Verification items for the finished model (mm, model axes). A direction names the side the tool comes from. Coordinates: 2 decimals unless noted, no trailing zeros. Order: outer loops, then holes, each group sorted by start corner. A loop starts at its lowest first (then second) coordinate and runs counter-clockwise, first axis right, second up. Notation, with made-up numbers: M 83,-19 L 121,-19 A21 cw 121,-7 Z; hole C -15,4.25 d8. An arc over 180 degrees is marked long. Return JSON: item names as keys, results as strings.
```python
from build123d import *

# Parameters (mm, degrees)
BOSS_EXTRUDE1_DEPTH = 5
FILLET1_R           = 10
BOSS_EXTRUDE2_DEPTH = 9.2
CUT_EXTRUDE1_DEPTH  = 3.2
SKETCH2_R           = 2.4999999999999996
SKETCH2_R_2         = 2.500000000000053
SKETCH2_R_3         = 2.5000000000000964
SKETCH2_R_4         = 2.5000000000000018
SKETCH2_R_5         = 2.4999999999999947
SKETCH2_R_6         = 14.287500000000001
CUT_EXTRUDE2_DEPTH  = 50.49730061393943
FILLET2_R           = 10


with BuildPart() as part:
    # Sketch1 → Boss-Extrude1 (new body)
    with BuildSketch(Plane(origin=(0, 0, 0), x_dir=(1, 0, 0), z_dir=(0, 1, 0))):
        Polygon((31.8, 18.359738560230117), (-9.39e-15, 36.719477120460205), (-31.799999999999994, 18.359738560230117), (-31.799999999999986, -18.359738560230095), (2.025e-14, -36.719477120460205), (31.800000000000008, -18.35973856023011), align=None)
    extrude(amount=BOSS_EXTRUDE1_DEPTH)

    # Fillet1
    fillet1_edges = [part.edges().sort_by_distance(p)[0] for p in [
        (31.800000000000008, 2.5, 18.35973856023011),
        (2.025e-14, 2.5, 36.719477120460205),
        (-31.799999999999986, 2.5, 18.359738560230095),
        (-31.799999999999994, 2.5, -18.359738560230117),
        (-9.39e-15, 2.5, -36.719477120460205),
        (31.8, 2.5, -18.359738560230117),
    ]]
    fillet(fillet1_edges, radius=FILLET1_R)

    # Sketch3 → Boss-Extrude2 (add)
    with BuildSketch(Plane.XZ):
        Polygon((27.499999999999996, 15.877132402714718), (9.57e-15, 31.754264805429415), (-27.500000000000004, 15.877132402714711), (-27.499999999999996, -15.877132402714711), (1.826e-14, -31.754264805429422), (27.50000000000001, -15.877132402714718), align=None)
    extrude(amount=BOSS_EXTRUDE2_DEPTH)

    # Sketch4 → Cut-Extrude1 (cut)
    with BuildSketch(Plane.XZ):
        Polygon((2.8499999999999854, -30.108816538239008), (4.199999999999984, -32.44708512845699), (26.000000000000007, -19.86084926012314), (24.650000000000006, -17.522580669905157), align=None)
        Polygon((-25.999999999999996, -19.860849260123146), (-4.200000000000003, -32.447085128456976), (-2.8499999999999983, -30.108816538238976), (-24.649999999999988, -17.52258066990515), align=None)
        Polygon((27.499999999999996, -12.586235868333851), (30.200000000000003, -12.586235868333851), (30.200000000000006, 12.586235868333848), (27.499999999999996, 12.586235868333848), align=None)
        Polygon((24.650000000000006, 17.522580669905146), (26.00000000000001, 19.860849260123135), (4.200000000000031, 32.44708512845697), (2.8500000000000263, 30.108816538238973), align=None)
        Polygon((-30.19999999999999, 12.58623586833384), (-30.199999999999996, -12.586235868333855), (-27.5, -12.58623586833386), (-27.500000000000004, 12.58623586833384), align=None)
        Polygon((-4.199999999999982, 32.44708512845697), (-25.99999999999999, 19.860849260123125), (-24.64999999999999, 17.52258066990515), (-2.849999999999986, 30.108816538238987), align=None)
    extrude(amount=-CUT_EXTRUDE1_DEPTH, mode=Mode.SUBTRACT)

    # Sketch2 → Cut-Extrude2 (cut, through all)
    with BuildSketch(Plane(origin=(0, 5, 0), x_dir=(1, 0, 0), z_dir=(0, 1, 0))):
        with Locations(Location((1.561e-14, 23.799999999999994, 0), (0, 0, 270))):
            Circle(SKETCH2_R)
        with Locations(Location((20.61140461006965, 11.899999999999997, 0), (0, 0, 270))):
            Circle(SKETCH2_R_2)
        with Locations(Location((20.61140461006965, -11.899999999999993, 0), (0, 0, 270))):
            Circle(SKETCH2_R_3)
        with Locations(Location((-1.561e-14, -23.800000000000015, 0), (0, 0, 270))):
            Circle(SKETCH2_R_4)
        with Locations(Location((-20.61140461006965, -11.899999999999993, 0), (0, 0, 270))):
            Circle(SKETCH2_R_5)
        with Locations(Location((-20.611404610069634, 11.899999999999999, 0), (0, 0, 270))):
            Circle(SKETCH2_R_5)
        with Locations(Location((0, 0, 0), (0, 0, 270))):
            Circle(SKETCH2_R_6)
    extrude(amount=-CUT_EXTRUDE2_DEPTH, mode=Mode.SUBTRACT)

    # Fillet2
    fillet2_edges = [part.edges().sort_by_distance(p)[0] for p in [
        (27.499999999999996, -4.6, 15.877132402714718),
        (9.57e-15, -4.6, 31.754264805429415),
        (-27.500000000000004, -4.6, 15.877132402714711),
        (-27.499999999999996, -4.6, -15.877132402714711),
        (27.50000000000001, -4.6, -15.877132402714718),
        (1.826e-14, -4.6, -31.754264805429422),
    ]]
    fillet(fillet2_edges, radius=FILLET2_R)


solid = part.part
```
Q1. Cross-section at D-D, the plane y = -3.5. Record the boundary of the cut face in (x, z) (1 decimal), and give its area (3 significant figures).
Values:
{"outline": "M -27.5,-10.1 A10 ccw -22.5,-18.8 L -5,-28.9 A10 ccw 5,-28.9 L 22.5,-18.8 A10 ccw 27.5,-10.1 L 27.5,10.1 A10 ccw 22.5,18.8 L 5,28.9 A10 ccw -5,28.9 L -22.5,18.8 A10 ccw -27.5,10.1 Z; hole C -20.6,-11.9 d5; hole C -20.6,11.9 d5; hole C 0,0 d28.6; hole C 0,-23.8 d5; hole C 0,23.8 d5; hole C 20.6,-11.9 d5; hole C 20.6,11.9 d5", "area": "1,830 mm^2"}
Q2. Cross-section at A-A, the plane x = 0. Record the boundary of the cut face in (y, z).
Values:
{"outline": "M -9.2,-30.21 L 0,-30.21 L 0,-35.17 L 5,-35.17 L 5,-26.3 L -9.2,-26.3 Z; M -9.2,-21.3 L 5,-21.3 L 5,-14.29 L -9.2,-14.29 Z; M -9.2,14.29 L 5,14.29 L 5,21.3 L -9.2,21.3 Z; M -9.2,26.3 L 5,26.3 L 5,35.17 L 0,35.17 L 0,30.21 L -9.2,30.21 Z"}
Q3. Material ranges on line 1 along X through (y, z) = (-4.25, -11.9); line 2 along Z through (x, y) = (-1, 2.5); line 3 along X through (y, z) = (-6.5, 0), recorded low to high.
Values:
{"line 1": "-27.34 to -23.11, -18.11 to -7.91, 7.91 to 18.11, 23.11 to 27.34", "line 2": "-35.12 to -26.09, -21.51 to -14.25, 14.25 to 21.51, 26.09 to 35.12", "line 3": "-27.5 to -14.29, 14.29 to 27.5"}
Q4. Go/stop test with flat-tipped pins: pin 1 (8 mm diameter, centred on y = 1.5, z = -27.5, fed in from +X); pin 2 (6 mm diameter, centred on x = -16, z = -27, fed in from -Y); pin 3 (4 mm diameter, centred on x = 25.5, y = 2, fed in from +Z). Record where each tip stops, or that it passes through.
Values:
{"pin 1": "x = 22.9", "pin 2": "y = 0", "pin 3": "z = 23.15"}
Q5. Cross-section at C-C, the plane x = -13. Record the boundary of the cut face in (y, z).
Values:
{"outline": "M -9.2,-24.25 L 3.2,-24.25 L 3.2,-27.37 L 0,-27.37 L 0,-29.21 L 5,-29.21 L 5,-5.93 L -9.2,-5.93 Z; M -9.2,5.93 L 5,5.93 L 5,29.21 L 0,29.21 L 0,27.37 L 3.2,27.37 L 3.2,24.25 L -9.2,24.25 Z"}
Q6. Draft check along Z on faces 3 (the face through (-14, 3.2, 25)), 4 (the face through (16.053, 2.465, -27.452)), 5 (the face through (15.747, 2.465, 27.628)). Enter one of: pulls with the +Z half, pulls with the -Z half, needs draft (parallel to the pull), parting line crosses it, or undercut.
Values:
{"face 3": "undercut", "face 4": "pulls with the -Z half", "face 5": "pulls with the +Z half"}
Q7. Cross-section at B-B, the plane z = 0. Record the boundary of the cut face in (x, y), and give its area (3 significant figures).
Values:
{"outline": "M -31.8,0 L -30.2,0 L -30.2,3.2 L -27.5,3.2 L -27.5,-9.2 L -14.29,-9.2 L -14.29,5 L -31.8,5 Z; M 14.29,-9.2 L 27.5,-9.2 L 27.5,3.2 L 30.2,3.2 L 30.2,0 L 31.8,0 L 31.8,5 L 14.29,5 Z", "area": "401 mm^2"}
Q8. Tool access check on faces 1 (the face through (-15.253, 1.578, -26.066)), 2 (the face through (-18.133, -2.001, 11.575)). Record the directions out of +Z, -Z, +X, -X, +Y, -Y that give a thin tool (end or side, any length) a straight path to the whole face; none if there is none.
Values:
{"face 1": "-Y", "face 2": "+Y, -Y"}
